Part model, mm, in its own coordinate system. Face numbers are marked on the shaded views. A direction names the side the tool comes from. Round coordinates to 2 decimals unless told otherwise and drop trailing zeros. Write each loop counter-clockwise with the first axis right and the second up, starting at its lowest first coordinate (ties: lowest second). Pieces come first, ordered by that corner, then holes. Notation, with made-up numbers: M 48,3.5 L 58,3.5 A22 cw 58,30.5 Z; hole C 16,26 d10. An arc over 180 degrees is marked long. Use one line per item in the form item = value. Start each with the question number.
Item 1: Mould opens along X. For the marked faces 3 and 4 say: +X half, -X half, draft (parallel to the pull), parting line (faces both ways), or undercut.
Item 2: Which spindle directions (+Z, -Z, +X, -X, +Y, -Y) get a long thin tool onto all of the face, cutting with end or side? Do the marked faces 1 and 2. Say none if no direction does.
Item 3: Cut at D-D, the plane y = 13.5. Give the cut face in (x, z).
Item 4: Cut at B-B, the plane y = -9.5. Give the cut face in (x, z), then the cut area to 3 significant figures.
Item 5: Cut at C-C, the plane z = 14.25. State how many separate pieces and enclosed holes the cut face has, then the cut area to 3 significant figures.
Item 6: Cut at A-A, the plane z = 17.25. Give the cut face in (x, y), then the cut area to 3 significant figures.
Item 7: Flat gauge pins, fed straight in: pin 1 Ø1 at (x, y) = (-9.5, 0) entering from -Z; pin 2 Ø1 at (x, y) = (-9.5, 7.5) entering from +Z; pin 3 Ø3 at (x, y) = (-5, 4.5) entering from +Z. Where does each tip first touch, or does it go through?
Item 8: Probe L1, parallel to Y at x = 0, z = 11.4; L2, parallel to Y at x = 0, z = 13.6; L3, parallel to Y at x = 3.5, z = 10.5. List the from-to ranges inside material, lowest first.
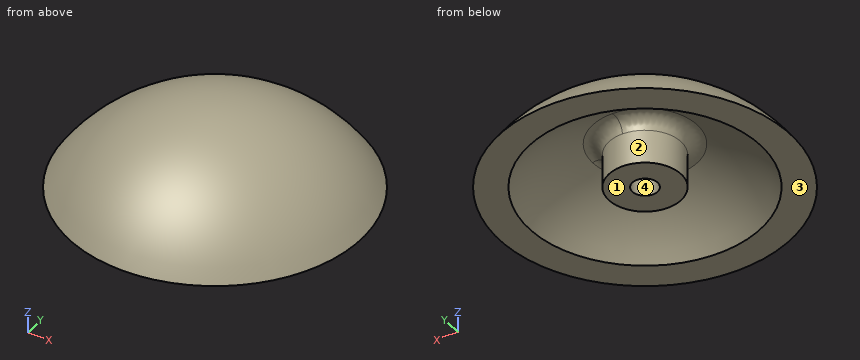
from build123d import *

# Parameters (mm, degrees)
F3_T     = -2.54
F4_R     = 3.81
F4_R_2   = 1.3335
F6_R     = 1.27
F7_R     = 18.415
F8_DEPTH = 10.16


with BuildPart() as f2:
    # F1 (on Right) → F2 (revolve)
    with BuildSketch(Plane.YZ):
        with BuildLine():
            Line((0, 18.415), (0, 0))
            Line((0, 0), (18.415, 0))
            ThreePointArc((18.415, 0), (13.0213713756, 13.0213713756), (0, 18.415))
        make_face()
    revolve(axis=Axis((0, 0, 9.2075), (0, 0, 1)))

    # F3
    f3_openings = [f2.faces().sort_by_distance(p)[0] for p in [
        (0, 0, 0),
    ]]
    offset(amount=F3_T, openings=f3_openings)

    # F4 (on face) → F5 (join, up to the next surface of F2)
    with BuildSketch(Plane.XY):
        Circle(F4_R)
        Circle(F4_R_2, mode=Mode.SUBTRACT)
    extrude(until=Until.NEXT)

    # F6
    f6_edges = [f2.edges().sort_by_distance(p)[0] for p in [
        (-2.694077, -2.694077, 15.41102),
        (2.694077, 2.694077, 15.41102),
    ]]
    fillet(f6_edges, radius=F6_R)

    # F7 (on face) → F8 (cut)
    with BuildSketch(Plane.XY):
        Circle(F7_R)
    extrude(amount=F8_DEPTH, mode=Mode.SUBTRACT)


solid = f2.part
Model answer:
q1.face_3 = draft
q1.face_4 = undercut
q2.face_1 = -Z, +X, -X, +Y, -Y
q2.face_2 = -Z
q3.outline = M -7.32,10.16 L 7.32,10.16 A12.52 ccw Z
q4.outline = M -12.07,10.16 L -7.65,10.16 A12.72 cw 7.65,10.16 L 12.07,10.16 A15.78 ccw Z
q4.area = 67.5 mm²
q5.separate_pieces = 2
q5.enclosed_holes = 2
q5.area = 317 mm²
q6.outline = C 0,0 d12.89
q6.area = 131 mm²
q7.pin_1 = 12.33
q7.pin_2 = 14.3
q7.pin_3 = 17.66
q8.L1 = -14.46 to -11.05, -3.81 to -1.33, 1.33 to 3.81, 11.05 to 14.46
q8.L2 = -12.42 to -8.19, -3.81 to -1.33, 1.33 to 3.81, 8.19 to 12.42
q8.L3 = -14.72 to -11.38, -1.51 to 1.51, 11.38 to 14.72
